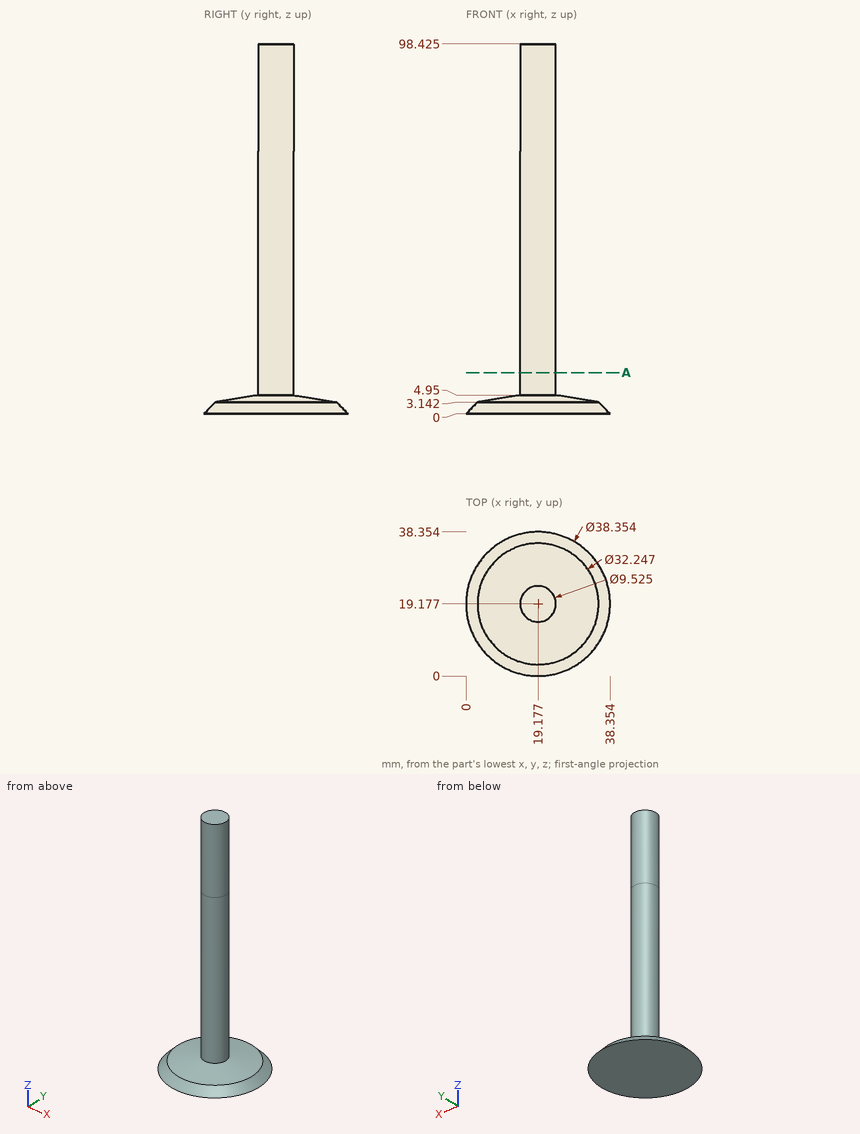
Geometry: see drawing. Coordinates: mm, zero at the bounding-box minimum. Round coordinates to 2 decimals unless told otherwise and drop trailing zeros. Loops run counter-clockwise (first coordinate to the right, second up) from the corner with the lowest first, then second, coordinate; pieces in that order, holes last. Notation, with made-up numbers: M 10.5,60 L 66.5,60 A25 cw 66.5,76 Z; hole C 52,76 d11. An arc over 180 degrees is marked long. Use a Markdown table: item, result. Add a question column.
1. Cut plane A-A, the plane z = 11. Output: boundary loops of the cut face in (x, y) (1 decimal).
2. Ray query, line 1 along X through (y, z) = (19, 60.5); line 2 along Y through (x, z) = (17.5, 18) (1 decimal); line 3 along Z through (x, y) = (31.5, 22). Return the intervals inside material, ascending. Write a range as [from, to].
3. Contact query for flat-ended pins moving along their axis: pin 1 (6 mm diameter, centred on x = 28.5, y = 29.5, fed in from +Z); pin 2 (10 mm diameter, centred on y = 17, z = 77.5, fed in from -X). Output: stop coordinate, or through.
Solution:
| question | item | result |
|---|---|---|
| 1 | outline | C 19.2,19.2 d9.5 |
| 2 | line 1 | x = [14.42, 23.94] |
| 2 | line 2 | y = [14.7, 23.6] |
| 2 | line 3 | z = [0, 3.7] |
| 3 | pin 1 | stops at z = 3.97 |
| 3 | pin 2 | stops at x = 14.41 |
